Here's how the part is built. I have some questions about the finished solid (model axes, mm). Round coordinates to 2 decimals unless told otherwise and drop trailing zeros. Loops run counter-clockwise (first coordinate to the right, second up) from the corner with the lowest first, then second, coordinate; pieces in that order, holes last. Notation, with made-up numbers: M 19,21.25 L 27,21.25 A21 cw 27,42.25 Z; hole C -40,51.5 d7. An arc over 180 degrees is marked long. Answer as CSV lines item,"result".
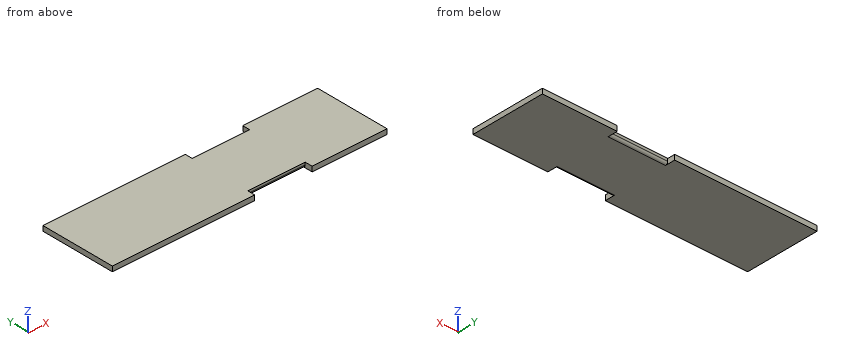
```python
from build123d import *

# Parameters (mm, degrees)
F0_W     = 110
F0_H     = 30
F1_DEPTH = 2
F2_W     = 23
F2_H     = 3
F3_DEPTH = 25
F4_R     = 1


with BuildPart() as f1:
    # F0 (on Top) → F1 (new body)
    with BuildSketch(Plane.XY):
        Rectangle(F0_W, F0_H)
    extrude(amount=F1_DEPTH)

    # F2 (on face) → F3 (cut)
    with BuildSketch(Plane.XY.offset(2)):
        with Locations((13.5, 13.5)):
            Rectangle(F2_W, F2_H)
        with Locations((13.5, -13.5)):
            Rectangle(F2_W, F2_H)
    extrude(amount=-F3_DEPTH, mode=Mode.SUBTRACT)

    # F4
    f4_edges = [f1.edges().sort_by_distance(p)[0] for p in [
        (13.5, -12, 0),
        (13.5, 12, 0),
    ]]
    fillet(f4_edges, radius=F4_R)


solid = f1.part
```
1. I want a section at B-B, the plane z = 1.4. Please give me the cut outline in (x, y), and give its area (3 significant figures).
Evaluation:
outline,"M -55,-15 L 2,-15 L 2,-12 L 25,-12 L 25,-15 L 55,-15 L 55,15 L 25,15 L 25,12 L 2,12 L 2,15 L -55,15 Z"
area,"3,160 mm²"
2. I want a section at C-C, the plane x = 21. Please give me the cut outline in (y, z), and give its area (3 significant figures).
Evaluation:
outline,"M -12,1 A1 ccw -11,0 L 11,0 A1 ccw 12,1 L 12,2 L -12,2 Z"
area,"47.6 mm²"
3. For P1, Ø0.5, axis at x = 8, z = 1.5, coming from the -Y side; P2, Ø0.8, axis at x = 12.5, z = 1.5, coming from the +Y side, each with a flat end and sliding along its axis, tell me the tip position at first contact or that it passes through.
Evaluation:
P1,"stops at y = -12"
P2,"stops at y = 12"
4. If I drill on line 1 (X direction, y = 12.5, z = 1.3); line 2 (Y direction, x = 4, z = 1.25); line 3 (Y direction, x = 8, z = 0.4), over which ranges is the centre line in solid material (lowest first)? Write a range as [from, to].
Evaluation:
line 1,"x = [-55, 2], [25, 55]"
line 2,"y = [-12, 12]"
line 3,"y = [-11.8, 11.8]"
5. I want a section at A-A, the plane y = -13. Please give me the cut outline in (x, z).
Evaluation:
outline,"M -55,0 L 2,0 L 2,2 L -55,2 Z; M 25,0 L 55,0 L 55,2 L 25,2 Z"
